The drawing under review shows one solid part. Ordinate dimensions are in mm from its lowest x, y, z. Round coordinates to 2 decimals unless told otherwise and drop trailing zeros. Write each loop counter-clockwise with the first axis right and the second up, starting at its lowest first coordinate (ties: lowest second). Pieces come first, ordered by that corner, then holes. Notation, with made-up numbers: M 68.5,75 L 104.5,75 A27 ccw 104.5,107 Z; hole C 19,-22 d9. An arc over 180 degrees is marked long. Write item = value, one per line. Start each with the question number.
Item 1: Take a section at C-C, the plane y = 27. Give the boundary of the cut face in (x, z), plus the area to 3 significant figures.
Item 2: Take a section at A-A, the plane z = 4.25. Give the boundary of the cut face in (x, y).
Item 3: For pin 1 Ø11.5 at (x, y) = (66, 13) entering from +Z, flat-tipped, find the tip position at first contact; note if it passes through.
Item 4: Take a section at B-B, the plane x = 21. Give the boundary of the cut face in (y, z), plus the area to 3 significant figures.
Item 5: The part is to be moulded in two halves that separate along Y. For the marked faces 1, 2, 3 and 4, say which applies: +Y half, -Y half, draft (parallel to the pull), parting line (faces both ways), or undercut.
Item 6: To check wall thickness, follow line 1 along Y through (x, z) = (28, 11.25); line 2 along X through (y, z) = (35.5, 11.5); line 3 along Z through (x, y) = (86, 18.5). State the ranges of each line that lie inside material, in increasing order.
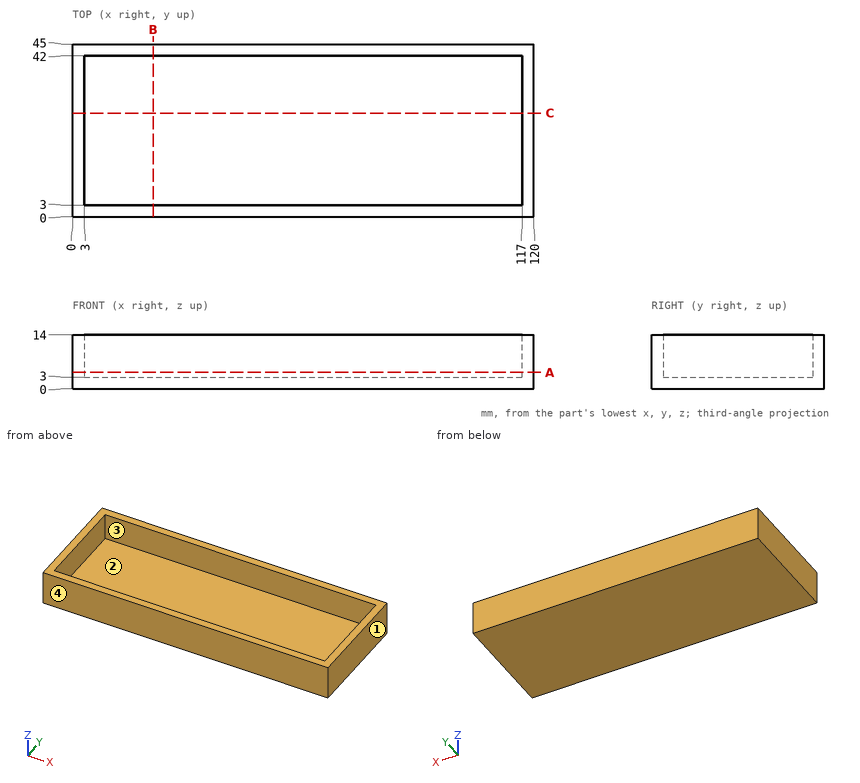
Response values:
q1.outline = M 0,0 L 120,0 L 120,14 L 117,14 L 117,3 L 3,3 L 3,14 L 0,14 Z
q1.area = 426 mm2
q2.outline = M 0,0 L 120,0 L 120,45 L 0,45 Z; hole M 3,3 L 117,3 L 117,42 L 3,42 Z
q3.pin_1 = 3
q4.outline = M 0,0 L 45,0 L 45,14 L 42,14 L 42,3 L 3,3 L 3,14 L 0,14 Z
q4.area = 201 mm2
q5.face_1 = draft
q5.face_2 = undercut
q5.face_3 = undercut
q5.face_4 = -Y half
q6.line_1 = 0 to 3, 42 to 45
q6.line_2 = 0 to 3, 117 to 120
q6.line_3 = 0 to 3
